Autodesk Inventor part; units mm, degrees
ref_plane "YZ Plane" through (0, 0, 0) normal (1, 0, 0) x (0, 1, 0)
ref_plane "XZ Plane" through (0, 0, 0) normal (0, 1, 0) x (-1, 0, 0)
ref_plane "XY Plane" through (0, 0, 0) normal (0, 0, 1) x (1, 0, 0)
sketch "草圖1" plane through (0, 0, 0) normal (0, 1, 0) x (-1, 0, 0)
  circle A0 centre (0, 0) radius 4
  dimension "d0" = 8
extrude "擠出1" add sketch "草圖1" along normal blind 1
sketch "草圖2" plane through (0, 1, 0) normal (0, 1, 0) x (1, 0, 0)
  circle A0 centre (0, 0) radius 4
  line L0 (2.3094, 4) -> (4.6188, 0)
  line L1 (4.6188, 0) -> (2.3094, -4)
  line L2 (2.3094, -4) -> (-2.3094, -4)
  line L3 (-2.3094, -4) -> (-4.6188, 0)
  line L4 (-4.6188, 0) -> (-2.3094, 4)
  line L5 (-2.3094, 4) -> (2.3094, 4)
  point P0 (0, 4)
extrude "擠出2" add sketch "草圖2" along normal blind 5
sketch "草圖3" plane through (0, 6, 0) normal (0, 1, 0) x (1, 0, 0)
  circle A0 centre (0, 0) radius 4
  dimension "d49" = 8
extrude "擠出3" add sketch "草圖3" along normal blind 6.5
fillet "圓角1" radius 1 1 edges at (-4, 12.5, 0)
sketch "草圖4" plane through (0, 12.5, 0) normal (0, 1, 0) x (1, 0, 0)
  circle A0 centre (0, 0) radius 3
  circle A1 centre (0, 0) radius 3
extrude "擠出4" add sketch "草圖4" along normal blind 1
sketch "草圖5" plane through (0, 13.5, 0) normal (0, 1, 0) x (1, 0, 0)
  circle A0 centre (0, 0) radius 3
  circle A1 centre (0, 0) radius 4
  dimension "d11" = 8
extrude "擠出5" add sketch "草圖5" along normal blind 1 contours A0 | A1
fillet "圓角2" radius 0.25 6 edges at (4.6188, 3.5, 0) (2.3094, 3.5, 4) (2.3094, 3.5, -4) (-2.3094, 3.5, -4) (-4.6188, 3.5, 0) (-2.3094, 3.5, 4)
sketch "草圖9" plane through (0, 0, 0) normal (0, 0, 1) x (1, 0, 0)
  line L0 (-4.75, 6) -> (-4, 6)
  line L1 (-4.75, 1) -> (-4, 1)
  line L2 (-4.75, 6) -> (-4.75, 5.5)
  line L3 (-4.75, 1) -> (-4.75, 1.5)
  arc A0 (-4, 6) -> (-4.75, 5.5) centre (-4, 5.1875) ccw
  arc A1 (-4.75, 1.5) -> (-4, 1) centre (-4, 1.8125) ccw
  line L4 (0, 0) -> (0, 9)
  dimension "d39" = 1
  dimension "d40" = 5
  dimension "d41" = 4
  dimension "d42" = 4
  dimension "d43" = 0.75
  dimension "d44" = 0.75
  dimension "d45" = 0.5
  dimension "d46" = 0.5
revolve "迴轉1" cut sketch "草圖9" angle 360 about axis through (0, 0, 0) along (0, 1, 0)
sketch "草圖10" plane through (0, 0, 0) normal (0, -1, 0) x (1, 0, 0)
  circle A0 centre (0, 0) radius 4
  circle A1 centre (0, 0) radius 3
  dimension "d54" = 6
extrude "擠出6" add sketch "草圖10" along normal blind 4 contours A1
thread "螺紋2"
sketch "草圖11" plane through (0, 14.5, 0) normal (0, 1, 0) x (1, 0, 0)
  circle A0 centre (0, 0) radius 4
hole "孔4" at (0, 14.5, 0) direction (0, -1, 0) diameter 2 end through all counterbore diameter 4 counterbore depth 10
chamfer "倒角1" distance 0.25 angle 45 2 edges at (-3, -4, 0) (0, -4, -1)
properties part number "pc4_m10"
Check sheet for the modelled part. Datum: model origin and axes. Units: mm. A direction names the side the tool comes from. Coordinates: 2 decimals unless noted, no trailing zeros. Write each loop counter-clockwise with the first axis right and the second up, starting at its lowest first coordinate (ties: lowest second). Pieces come first, ordered by that corner, then holes.
Item 1: Depth check by flat-ended pin: pin 1 Ø1 at (y, z) = (5.5, -1.5) entering from -X; pin 2 Ø1 at (y, z) = (10.5, 2.5) entering from -X; pin 3 Ø1.2 at (x, z) = (-1, 0.5) entering from +Y. Enter the tip coordinate at first touch or a pass-through.
Numbers:
pin 1: stops at x = -4.04
pin 2: stops at x = -3.46
pin 3: stops at y = 4.5
Item 2: Cross-section at B-B on y = -1.5. Record the boundary of the cut face in (x, z), then the cut area to 3 significant figures.
Numbers:
outline: circle Ø6 at (0, 0); hole circle Ø2 at (0, 0)
area: 25.1 mm2
Item 3: Cross-section at A-A on y = 10.5. Record the boundary of the cut face in (x, z), then the cut area to 3 significant figures.
Numbers:
outline: circle Ø8 at (0, 0); hole circle Ø4 at (0, 0)
area: 37.7 mm2
Item 4: Scan lines: probe 1 along X at (y, z) = (2, 0); probe 2 along X at (y, z) = (9, 0); probe 3 along Z at (x, y) = (0, -0.75). Record each from-to range of solid material in increasing order.
Numbers:
probe 1: x = -4.58 to -1, 1 to 4.58
probe 2: x = -4 to -2, 2 to 4
probe 3: z = -3 to -1, 1 to 3
Item 5: Mould release check, pull along Y, two halves, no side actions. Record for faces 4 (the face through (0, 3, -4)), 5 (the face through (1, 13.5, -3)), 6 (the face through (-2, 14.5, 1)): released by +Y, released by -Y, zero draft, split by the parting line, or undercut.
Numbers:
face 4: zero draft
face 5: undercut
face 6: released by +Y
Item 6: Access from +Z, -Z, +X, -X, +Y, -Y to the whole of each face (thin tool, end or side, straight path). Record for faces 1 (the face through (-0.867, 13.993, -3.905)), 2 (the face through (0.867, 0.493, 3.905)), 3 (the face through (-3, 13, 0)).
Numbers:
face 1: +Y
face 2: -Y
face 3: none
